Work out the finished part from the listing and answer in its coordinate system (mm). A direction names the side the tool comes from. Round coordinates to 2 decimals unless told otherwise and drop trailing zeros. Write each loop counter-clockwise with the first axis right and the second up, starting at its lowest first coordinate (ties: lowest second). Pieces come first, ordered by that corner, then holes. Notation, with made-up numbers: M 85.25,65 L 93.25,65 A14 cw 93.25,83 Z; hole C 83,14.5 d4. An arc over 180 degrees is marked long. One line per item, written item: value. Start each with the question number.
Q1. Find section C-C (z = 193). Write down the section's boundary in (x, y).
Q2. The mould has two halves that part along X. Classify faces 1 (the flat face through (-90.043, 7, 200)), 2 (the flat face through (88.519, 7, 200)), 3 (the flat face through (0, 1, 406.4)), 4 (the flat face through (90.043, 7, 200)): released by +X, released by -X, zero draft, split by the parting line, or undercut.
Q3. A tool of negligible diameter and unlimited length cuts with its end or side. For faces 5 (the flat face through (1, -8, -1.524)), 6 (the flat face through (-1, 0, 206)), 7 (the flat face through (1, 1.524, 206)), from which of +Z, -Z, +X, -X, +Y, -Y can it reach the whole face along a straight path? Write none if from no direction.
Q4. Find section B-B (x = 73.5). Write down the section's boundary in (y, z).
Q5. Given pin 1 Ø2.5 at (x, y) = (88, 3) entering from -Z; pin 2 Ø10 at (x, z) = (62, 131.5) entering from -Y; pin 3 Ø4 at (x, y) = (-10.5, -24.5) entering from -Z; pin 4 Ø4 at (y, z) = (-1, 349.5) entering from -X, each flat-ended and moving along its own axis, determine where each tip first touches the part or whether it passes through.
Q6. Consider probe 1 along Z at (x, y) = (-89, 6); probe 2 along Y at (x, z) = (88.8, 330.2); probe 3 along Y at (x, z) = (-89.55, 203.2). Determine where each line is inside the solid, lowest interval first.
Q7. Find section A-A (y = -19). Write down the section's boundary in (x, z).
from build123d import *

# Parameters (mm, degrees)
F0_W     = 180.086
F0_H     = 406.4
F1_DEPTH = 12.7
F2_T     = -1.524
F3_R     = 2
F4_DEPTH = 180.087
F5_W     = 173.736
F5_H     = 1.524
F6_DEPTH = 31.75
F8_DEPTH = 25.4
F9_R     = 1.27
F10_R    = 0.508


with BuildPart() as f1:
    # F0 (on Front) → F1 (new body)
    with BuildSketch(Plane.XZ):
        with Locations((0, 203.2)):
            Rectangle(F0_W, F0_H)
    extrude(amount=-F1_DEPTH)

    # F2
    f2_openings = [f1.faces().sort_by_distance(p)[0] for p in [
        (0, 6.35, 406.4),
        (0, 6.35, 0),
        (0, 12.7, 203.2),
    ]]
    offset(amount=F2_T, openings=f2_openings)

    # F3 (on face) → F4 (cut, through all)
    with BuildSketch(Plane.YZ.offset(90.043)):
        with Locations((6.35, 76.2)):
            Circle(F3_R)
        with Locations((6.35, 330.2)):
            Circle(F3_R)
        with Locations((6.35, 203.2)):
            Circle(F3_R)
    extrude(amount=-F4_DEPTH, mode=Mode.SUBTRACT)

    # F5 (on face) → F6 (join)
    with BuildSketch(Plane(origin=(0, 1.524, 0), x_dir=(-1, 0, 0), z_dir=(0, 1, 0))):
        with Locations((0, -0.762)):
            Rectangle(F5_W, F5_H)
    extrude(amount=-F6_DEPTH)

    # F7 (on face) → F8 (cut)
    with BuildSketch(Plane(origin=(0, 0, -1.524), x_dir=(1, 0, 0), z_dir=(0, 0, -1))):
        with BuildLine():
            ThreePointArc((-10.9985226281, 30.226), (-3.2870018728, 11.6087420061), (12.7, 23.876))
            ThreePointArc((12.7, 23.876), (12.2672579939, 27.1630018728), (10.9985226281, 30.226))
            Line((10.9985226281, 30.226), (-10.9985226281, 30.226))
        make_face()
    extrude(amount=-F8_DEPTH, mode=Mode.SUBTRACT)

    # F9
    f9_edges = [f1.edges().sort_by_distance(p)[0] for p in [
        (90.043, 0, 203.2),
        (0, 1.524, -1.524),
        (-90.043, 0, 203.2),
        (-10.998523, -30.226, -0.762),
        (10.998523, -30.226, -0.762),
        (-86.868, -30.226, -0.762),
        (86.868, -30.226, -0.762),
        (-89.281, 12.7, 0),
        (89.281, 12.7, 0),
        (89.281, 12.7, 406.4),
        (-89.281, 12.7, 406.4),
    ]]
    fillet(f9_edges, radius=F9_R)

    # F10
    f10_edges = [f1.edges().sort_by_distance(p)[0] for p in [
        (-88.519, 1.524, 203.2),
        (88.519, 1.524, 203.2),
        (0, 0, 0),
    ]]
    fillet(f10_edges, radius=F10_R)


solid = f1.part
The answers:
1. outline: M -90.04,1.27 A1.27 ccw -88.77,0 L 88.77,0 A1.27 ccw 90.04,1.27 L 90.04,12.7 L 88.52,12.7 L 88.52,2.03 A0.51 cw 88.01,1.52 L -88.01,1.52 A0.51 cw -88.52,2.03 L -88.52,12.7 L -90.04,12.7 Z
2. face 1: released by -X
2. face 2: undercut
2. face 3: zero draft
2. face 4: released by +X
3. face 5: -Z, +X, -X, +Y, -Y
3. face 6: +Z, +X, -X, -Y
3. face 7: +Z, -Z, +Y
4. outline: M -30.23,-1.52 L 0.25,-1.52 A1.27 ccw 1.52,-0.25 L 1.52,406.4 L 0,406.4 L 0,0.51 A0.51 cw -0.51,0 L -30.23,0 Z
5. pin 1: z = 0
5. pin 2: y = 0
5. pin 3: through
5. pin 4: x = -90.01
6. probe 1: 0 to 74.23, 78.17 to 201.23, 205.17 to 328.23, 332.17 to 406.4
6. probe 2: 0 to 4.35, 8.35 to 12.7
6. probe 3: 0.27 to 4.35, 8.35 to 12.7
7. outline: M -86.87,-1.52 L -11.73,-1.52 L -11.73,0 L -86.87,0 Z; M 11.73,-1.52 L 86.87,-1.52 L 86.87,0 L 11.73,0 Z
